Build history of the part. All positions in model axes, mm. A direction names the side the tool comes from. Give positions to 0.01 mm unless a question says otherwise; leave off trailing zeros. Loops run counter-clockwise (first coordinate to the right, second up) from the corner with the lowest first, then second, coordinate; pieces in that order, holes last. Notation, with made-up numbers: M 73.25,52 L 122.25,52 A15 cw 122.25,67 Z; hole C 55,57.5 d6. An arc over 180 degrees is marked long. Answer as a JSON object with one key per item and string values. Group by question number.
1. Drill centre lines: line 1 along Z through (x, y) = (-4, -3.75); line 2 along Z through (x, y) = (3.5, -9); line 3 along Y through (x, z) = (0.5, -6.5). Where is each one in solid material? Low to high. Write a range as [from, to].
2. Drop flat-ended pins along their axis: pin 1 Ø1 at (y, z) = (-8.5, -27.5) entering from -X; pin 2 Ø3 at (x, z) = (0, 13.5) entering from +Y; pin 3 Ø2 at (y, z) = (2, -3) entering from +X. Give the stop position or say it passes through.
3. Mould opens along X. For faces 1 (the face through (0, 0, -53.6)), 2 (the face through (-6.191, -7.145, -2.028)), 3 (the face through (-1.2, -1.6, 9.9)) say: released by +X, released by -X, zero draft, split by the parting line, or undercut.
4. Slice it at C-C (z = 9.5). List the corners of the cut face in (x, y).
5. Slice it at A-A (y = 0). List the corners of the cut face in (x, z).
6. 3-axis set-ups, long thin cutter, end or side, ignore diameter. For faces 4 (the face through (0, 0, 17.7)), 5 (the face through (5.6, 6.6, -2)), 6 (the face through (0, 1, 12)): which of +Z, -Z, +X, -X, +Y, -Y reach the whole face in a straight line?
7. Slice it at B-B (x = 0). List the corners of the cut face in (y, z).
8. Slice it at D-D (z = -23.5). List the corners of the cut face in (x, y), then the cut area to 3 significant figures.
from build123d import *

# Parameters (mm, degrees)
CUT_EXTRUDE1_DEPTH              = 11.3
TAP_DRILL_FOR_M2X0_4_TAP1_D     = 1.6
TAP_DRILL_FOR_M2X0_4_TAP1_DEPTH = 4
TAP_DRILL_FOR_M2X0_4_TAP1_TIP   = 0.480688495


with BuildPart() as part:
    # Sketch4 → Revolve1 (revolve)
    with BuildSketch(Plane(origin=(0, 0, 0), x_dir=(0, 0, -1), z_dir=(1, 0, 0))):
        Polygon((0, 8), (0, 11), (21.4, 11), (53.6, 11), (53.6, 0), (0, 0), (-17.7, 0), (-17.7, 2), (-2.4, 2), (-2.4, 8), align=None)
    revolve(axis=Axis((0, 0, 0), (0, 0, -1)))

    # Sketch5 → Cut-Extrude1 (cut)
    with BuildSketch(Plane.XY.offset(17.7)):
        with BuildLine():
            Line((1.732050808, 1), (-1.732050808, 1))
            ThreePointArc((-1.732050808, 1), (-1, 1.732050808), (0, 2))
            ThreePointArc((0, 2), (1, 1.732050808), (1.732050808, 1))
        make_face()
    extrude(amount=-CUT_EXTRUDE1_DEPTH, mode=Mode.SUBTRACT)

    # Tap Drill for M2x0.4 Tap1
    with Locations(Plane.XY):
        with Locations((6.363961031, 6.363961031), (6.363961031, -6.363961031), (-6.363961031, -6.363961031), (-6.363961031, 6.363961031)):
            Hole(TAP_DRILL_FOR_M2X0_4_TAP1_D / 2, depth=TAP_DRILL_FOR_M2X0_4_TAP1_DEPTH)
            with Locations((0, 0, -(TAP_DRILL_FOR_M2X0_4_TAP1_DEPTH + TAP_DRILL_FOR_M2X0_4_TAP1_TIP / 2))):  # 118° drill point
                Cone(0, TAP_DRILL_FOR_M2X0_4_TAP1_D / 2, TAP_DRILL_FOR_M2X0_4_TAP1_TIP, mode=Mode.SUBTRACT)


solid = part.part
Established:
{
 "1": {"line 1": "z = [-53.6, 2.4]", "line 2": "z = [-53.6, 0]", "line 3": "y = [-10.99, 10.99]"},
 "2": {"pin 1": "stops at x = -7.55", "pin 2": "stops at y = 1", "pin 3": "stops at x = 10.95"},
 "3": {"face 1": "zero draft", "face 2": "undercut", "face 3": "split by the parting line"},
 "4": {"outline": "M -1.73,1 A2 ccw long 1.73,1 Z"},
 "5": {"outline": "M -11,-53.6 L 11,-53.6 L 11,0 L 8,0 L 8,2.4 L 2,2.4 L 2,17.7 L -2,17.7 L -2,2.4 L -8,2.4 L -8,0 L -11,0 Z"},
 "6": {"face 4": "+Z, +X, -X, +Y, -Y", "face 5": "+Z", "face 6": "+Z, +X, -X, +Y"},
 "7": {"outline": "M -11,-53.6 L 11,-53.6 L 11,0 L 8,0 L 8,2.4 L 2,2.4 L 2,6.4 L 1,6.4 L 1,17.7 L -2,17.7 L -2,2.4 L -8,2.4 L -8,0 L -11,0 Z"},
 "8": {"outline": "C 0,0 d22", "area": "380 mm^2"}
}
